Here's how the part is built. I have some questions about the finished solid (model axes, mm). A direction names the side the tool comes from. Round coordinates to 2 decimals unless told otherwise and drop trailing zeros. Order: outer loops, then holes, each group sorted by start corner. A loop starts at its lowest first (then second) coordinate and runs counter-clockwise, first axis right, second up. Notation, with made-up numbers: (24, -4) - (65, -4) arc R13 ccw to (65, 1) - close; hole circle Ø7 at (32, 18.5). An arc over 180 degrees is marked (long way). Answer as a JSON object with one key per item and string values.
```python
from build123d import *
from OCP.BRepFilletAPI import BRepFilletAPI_MakeChamfer

# Parameters (mm, degrees)
BOSS_EXTRUDE1_DEPTH       = 38.6
BOSS_EXTRUDE1_DEPTH_BACK  = 38.6
BOSS_EXTRUDE2_DEPTH       = 25.25
BOSS_EXTRUDE2_DEPTH_BACK  = 25.25
CHAMFER1_SIZE             = 3
CHAMFER2_SIZE             = 2
CHAMFER2_SIZE2            = 2.828427125
FILLET1_R                 = 2
M6X1_0_TAPPED_HOLE1_D     = 5
M6X1_0_TAPPED_HOLE1_DEPTH = 25.981766235
M6X1_0_TAPPED_HOLE1_TIP   = 1.502151548
CHAMFER3_SIZE             = 1


with BuildPart() as part:
    # Sketch3 → Boss-Extrude1 (new, two sides: drawn at the far end of the back side and taken through both)
    with BuildSketch(Plane.XY.offset(-BOSS_EXTRUDE1_DEPTH_BACK)):
        Polygon((-21.518233765, 4.018233765), (-10.018233765, 4.018233765), (-6.55, 7.48646753), (-6.55, 10.41646753), (-10.018233765, 13.884701295), (-10.018233765, 15.214701295), (-7.16, 18), (7.16, 18), (10.018233765, 15.214701295), (10.018233765, 13.884701295), (6.55, 10.41646753), (6.55, 7.48646753), (10.018233765, 4.018233765), (21.518233765, 4.018233765), (21.518233765, 30), (-21.518233765, 30), align=None)
    extrude(amount=BOSS_EXTRUDE1_DEPTH + BOSS_EXTRUDE1_DEPTH_BACK)

    # Sketch3<4> → Boss-Extrude2 (add, two sides: drawn at the far end of the back side and taken through both)
    with BuildSketch(Plane.XY.offset(-BOSS_EXTRUDE2_DEPTH_BACK)):
        Polygon((-25.934509717, 20.5), (-21.518233765, 4.018233765), (-21.518233765, 30), (-31.5, 30), (-31.5, 20.5), align=None)
        Polygon((21.518233765, 30), (21.518233765, 4.018233765), (25.934509717, 20.5), (31.5, 20.5), (31.5, 30), align=None)
    extrude(amount=BOSS_EXTRUDE2_DEPTH + BOSS_EXTRUDE2_DEPTH_BACK)

    # Chamfer1
    chamfer1_edges = [part.edges().sort_by_distance(p)[0] for p in [
        (21.518233765, 4.018233765, -31.925),
        (-21.518233765, 4.018233765, -31.925),
        (-21.518233765, 4.018233765, 31.925),
        (21.518233765, 4.018233765, 31.925),
    ]]
    chamfer(chamfer1_edges, length=CHAMFER1_SIZE)

    # Chamfer2: one chamfer whose edges measure the first distance from different faces: ONE call of the kernel's chamfer builder (chamfer() names one face for all edges)
    chamfer2_edges_1 = [part.edges().sort_by_distance(p)[0] for p in [
        (-21.518233765, 4.018233765, 0),
    ]]
    chamfer2_side_1 = [part.faces().sort_by_distance(p)[0] for p in [
        (-15.346759208, 4.018233765, 0),
    ]]
    chamfer2_edges_2 = [part.edges().sort_by_distance(p)[0] for p in [
        (21.518233765, 4.018233765, 0),
    ]]
    chamfer2_side_2 = [part.faces().sort_by_distance(p)[0] for p in [
        (15.346759208, 4.018233765, 0),
    ]]
    chamfer2 = BRepFilletAPI_MakeChamfer(part.part.solid().wrapped)
    for e in chamfer2_edges_1:
        chamfer2.Add(CHAMFER2_SIZE, CHAMFER2_SIZE2, e.wrapped, chamfer2_side_1[0].wrapped)  # the first distance lies on this face
    for e in chamfer2_edges_2:
        chamfer2.Add(CHAMFER2_SIZE, CHAMFER2_SIZE2, e.wrapped, chamfer2_side_2[0].wrapped)  # the first distance lies on this face
    add(Compound.cast(chamfer2.Shape()), mode=Mode.REPLACE)

    # Fillet1
    fillet1_edges = [part.edges().sort_by_distance(p)[0] for p in [
        (-25.934509717, 20.5, 0),
        (25.934509717, 20.5, 0),
    ]]
    fillet(fillet1_edges, radius=FILLET1_R)

    # M6x1.0 Tapped Hole1
    with Locations(Plane(origin=(-26.5, 30, 20), x_dir=(0, 0, 1), z_dir=(0, 1, 0))):
        with Locations((0, 0), (-40, 0), (-40, 53), (0, 53)):
            Hole(M6X1_0_TAPPED_HOLE1_D / 2, depth=M6X1_0_TAPPED_HOLE1_DEPTH)
            with Locations((0, 0, -(M6X1_0_TAPPED_HOLE1_DEPTH + M6X1_0_TAPPED_HOLE1_TIP / 2))):  # 118° drill point
                Cone(0, M6X1_0_TAPPED_HOLE1_D / 2, M6X1_0_TAPPED_HOLE1_TIP, mode=Mode.SUBTRACT)

    # Chamfer3
    chamfer3_edges = [part.edges().sort_by_distance(p)[0] for p in [
        (31.5, 25.25, 25.25),
        (-31.5, 25.25, 25.25),
        (-31.5, 25.25, -25.25),
        (31.5, 25.25, -25.25),
    ]]
    chamfer(chamfer3_edges, length=CHAMFER3_SIZE)


solid = part.part
```
1. If I drill on L1, parallel to X at y = 23.25, z = -20; L2, parallel to Z at x = 26.5, y = 22.5; L3, parallel to Y at x = 6, z = -28, over which ranges is the centre line in solid material (lowest first)? Write a range as [from, to].
Responses:
{"L1": "[-31.5, -29], [-24, 24], [29, 31.5]", "L2": "[-25.25, -22.5], [-17.5, 17.5], [22.5, 25.25]", "L3": "[18, 30]"}
2. Thinking about a two-plate mould opening in Y: for faces 5 (the face through (-26.24, 20.08, 23.8)), 6 (the face through (6.55, 9, -1)), 7 (the face through (-8.609, 16.588, -0.54)), which applies, pulls with the +Y half, pulls with the -Y half, needs draft (parallel to the pull), parting line crosses it, or undercut?
Responses:
{"face 5": "pulls with the -Y half", "face 6": "needs draft", "face 7": "undercut"}
3. Imagine slicing it at B-B (x = 26.5). List the corners of the cut face in (y, z) for me.
Responses:
{"outline": "(20.25, -25.25) - (30, -25.25) - (30, -22.5) - (20.25, -22.5) - close; (20.25, -17.5) - (30, -17.5) - (30, 17.5) - (20.25, 17.5) - close; (20.25, 22.5) - (30, 22.5) - (30, 25.25) - (20.25, 25.25) - close"}
4. For faces 1 (the face through (21.518, 18, 32)), 2 (the face through (8.569, 16.627, -0.54)), 3 (the face through (-21.518, 19, -32)), 4 (the face through (-20, 5.5, -32)), which set-ups out of +Z, -Z, +X, -X, +Y, -Y let a thin tool reach every point of the face, with its end or its side?
Responses:
{"face 1": "+Z, +X, +Y, -Y", "face 2": "+Z, -Z", "face 3": "-Z, -X, +Y, -Y", "face 4": "-Z, -X, -Y"}
5. Imagine slicing it at C-C (y = 23.75). List the corners of the cut face in (x, z) for me.
Responses:
{"outline": "(-31.5, -24.25) - (-30.5, -25.25) - (-21.52, -25.25) - (-21.52, -38.6) - (21.52, -38.6) - (21.52, -25.25) - (30.5, -25.25) - (31.5, -24.25) - (31.5, 24.25) - (30.5, 25.25) - (21.52, 25.25) - (21.52, 38.6) - (-21.52, 38.6) - (-21.52, 25.25) - (-30.5, 25.25) - (-31.5, 24.25) - close; hole circle Ø5 at (-26.5, -20); hole circle Ø5 at (-26.5, 20); hole circle Ø5 at (26.5, -20); hole circle Ø5 at (26.5, 20)"}
6. Imagine slicing it at A-A (z = -20). List the corners of the cut face in (x, y) for me.
Responses:
{"outline": "(-31.5, 20.5) - (-29, 20.5) - (-29, 30) - (-31.5, 30) - close; (-24, 13.28) - (-22.25, 6.75) - (-19.52, 4.02) - (-10.02, 4.02) - (-6.55, 7.49) - (-6.55, 10.42) - (-10.02, 13.88) - (-10.02, 15.21) - (-7.16, 18) - (7.16, 18) - (10.02, 15.21) - (10.02, 13.88) - (6.55, 10.42) - (6.55, 7.49) - (10.02, 4.02) - (19.52, 4.02) - (22.25, 6.75) - (24, 13.28) - (24, 30) - (-24, 30) - close; (29, 20.5) - (31.5, 20.5) - (31.5, 30) - (29, 30) - close"}
7. For P1, Ø4.5, axis at x = -0.5, z = -9.5, coming from the -Y side; P2, Ø1, axis at y = 10.5, z = -10, coming from the +X side; P3, Ø4, axis at y = 23.5, z = 29.5, coming from the -X side; P4, Ø3.5, axis at x = -22, y = 19, coming from the -Z side, each with a flat end and sliding along its axis, tell me the tip position at first contact or that it passes through.
Responses:
{"P1": "y = 18", "P2": "x = 23.39", "P3": "x = -21.52", "P4": "z = -38.6"}
8. Imagine slicing it at D-D (z = 12). List the corners of the cut face in (x, y) for me.
Responses:
{"outline": "(-31.5, 20.5) - (-27.47, 20.5) arc R2 cw to (-25.54, 19.02) - (-22.25, 6.75) - (-19.52, 4.02) - (-10.02, 4.02) - (-6.55, 7.49) - (-6.55, 10.42) - (-10.02, 13.88) - (-10.02, 15.21) - (-7.16, 18) - (7.16, 18) - (10.02, 15.21) - (10.02, 13.88) - (6.55, 10.42) - (6.55, 7.49) - (10.02, 4.02) - (19.52, 4.02) - (22.25, 6.75) - (25.54, 19.02) arc R2 cw to (27.47, 20.5) - (31.5, 20.5) - (31.5, 30) - (-31.5, 30) - close"}
